```python
from build123d import *

# Parameters (mm, degrees)
F0_W     = 6.5
F0_H     = 9.5
F0_W_2   = 2
F0_H_2   = 13.4
F0_W_3   = 15.45
F0_H_3   = 16.4
F0_W_4   = 18.45
F0_H_4   = 0.8
F1_DEPTH = 1
F2_DEPTH = 3.5
F3_START = 3.5
F0_H_5   = 0.225
F3_DEPTH = 4.2
F4_DEPTH = 2.5


with BuildPart() as f1:
    # F0 (on Top) → F1 (new body)
    with BuildSketch(Plane.XY):
        with Locations((3.25, -9)):
            Rectangle(F0_W, F0_H)
        with Locations((43.5, -7.5)):
            Rectangle(F0_W_2, F0_H_2)
        Polygon((45, 0), (42.5, 0), (42.5, -0.8), (44.5, -0.8), (44.5, -14.2), (45, -14.2), align=None)
        with Locations((16.325, -9)):
            Rectangle(F0_W_3, F0_H_3)
        Polygon((42.5, -0.8), (24.05, -0.8), (24.05, -17.2), (42.5, -17.2), (42.5, -14.2), align=None)
        with Locations((33.275, -0.4)):
            Rectangle(F0_W_4, F0_H_4)
        Polygon((24.05, 0), (0, 0), (0, -4.25), (6.5, -4.25), (6.5, -13.75), (0, -13.75), (0, -18), (24.05, -18), (24.05, -17.2), (8.6, -17.2), (8.6, -0.8), (24.05, -0.8), align=None)
        with Locations((33.275, -17.6)):
            Rectangle(F0_W_4, F0_H_4)
    extrude(amount=F1_DEPTH)

    # F0 (on Top) → F2 (join)
    with BuildSketch(Plane.XY):
        with Locations((16.325, -9)):
            Rectangle(F0_W_3, F0_H_3)
        Polygon((42.5, -0.8), (24.05, -0.8), (24.05, -17.2), (42.5, -17.2), (42.5, -14.2), align=None)
        with Locations((43.5, -7.5)):
            Rectangle(F0_W_2, F0_H_2)
    extrude(amount=F2_DEPTH)

    # F0 (on Top) → F3 (join)
    with BuildSketch(Plane.XY.offset(F3_START)):
        with Locations((33.275, -0.4)):
            Rectangle(F0_W_4, F0_H_4)
        with Locations((33.275, 0.1125)):
            Rectangle(F0_W_4, F0_H_5)
        Polygon((42.5, -0.8), (24.05, -0.8), (24.05, -17.2), (42.5, -17.2), (42.5, -14.2), align=None)
        with Locations((33.275, -17.6)):
            Rectangle(F0_W_4, F0_H_4)
        with Locations((33.275, -18.1125)):
            Rectangle(F0_W_4, F0_H_5)
    extrude(amount=F3_DEPTH)

    # F0 (on Top) → F4 (join)
    with BuildSketch(Plane.XY):
        with Locations((3.25, -9)):
            Rectangle(F0_W, F0_H)
    extrude(amount=F4_DEPTH)


solid = f1.part
```
Geometry: final body of the model. Coordinates: model frame, mm. A direction names the side the tool comes from. Coordinates: 2 decimals unless noted, no trailing zeros. Order: outer loops, then holes, each group sorted by start corner. A loop starts at its lowest first (then second) coordinate and runs counter-clockwise, first axis right, second up. Notation, with made-up numbers: (51.5, 19) - (78.5, 19) arc R9 ccw to (78.5, 31) - close; hole circle Ø10 at (-2.5, -31). An arc over 180 degrees is marked (long way). Return JSON: item names as keys, results as strings. Group by question number.
1. Set-up query: faces 4 (the face through (3, -9, 2.5)), 5 (the face through (25, -17.2, 2)), 6 (the face through (44.5, -8, 2)), 7 (the face through (6.5, -9, 2)). Return all of +Z, -Z, +X, -X, +Y, -Y with unobstructed straight access to the full face (end or side cutting, diameter ignored); none if empty.
2. Cut plane D-D (z = 6). Output: boundary loops of the cut face in (x, y) (3 decimals), plus the area to 3 significant figures.
3. Material intervals for line 1 along X through (y, z) = (-8.75, 2.25); line 2 along Y through (x, z) = (13.5, 1.25); line 3 along X through (y, z) = (-16.5, 3.25), sorted ascending. Write a range as [from, to].
4. Pull-direction query (Z, two-part tool) for faces 1 (the face through (22, -9, 0)), 2 (the face through (7, -9, 1)), 3 (the face through (8.6, -9, 2)); classes: pulls with the +Z half, pulls with the -Z half, needs draft (parallel to the pull), parting line crosses it, or undercut.
5. Cut plane C-C (y = -13.25). Output: boundary loops of the cut face in (x, z), plus the area to 3 significant figures.
6. Pin query (flat end, axial travel): pin 1 (1.5 mm diameter, centred on y = -7, z = 6.5, fed in from -X); pin 2 (1 mm diameter, centred on x = 33, z = 2.5, fed in from +Y); pin 3 (5 mm diameter, centred on x = 2, y = -11, fed in from +Z). Return the tip coordinate at first contact, or that it passes through.
7. Cut plane B-B (x = 9). Output: boundary loops of the cut face in (y, z).
8. Cut plane A-A (z = 2). Output: boundary loops of the cut face in (x, y), plus the area to 3 significant figures.
Resolved:
{
 "1": {"face 4": "+Z, -X, +Y, -Y", "face 5": "+X, -X, -Y", "face 6": "+Z, +X, +Y, -Y", "face 7": "+Z, +Y, -Y"},
 "2": {"outline": "(24.05, -18.225) - (42.5, -18.225) - (42.5, 0.225) - (24.05, 0.225) - close", "area": "340 mm²"},
 "3": {"line 1": "x = [0, 6.5], [8.6, 44.5]", "line 2": "y = [-17.2, -0.8]", "line 3": "x = [8.6, 42.5]"},
 "4": {"face 1": "pulls with the -Z half", "face 2": "undercut", "face 3": "needs draft"},
 "5": {"outline": "(0, 0) - (45, 0) - (45, 1) - (44.5, 1) - (44.5, 3.5) - (42.5, 3.5) - (42.5, 7.7) - (24.05, 7.7) - (24.05, 3.5) - (8.6, 3.5) - (8.6, 1) - (6.5, 1) - (6.5, 2.5) - (0, 2.5) - close", "area": "222 mm²"},
 "6": {"pin 1": "stops at x = 24.05", "pin 2": "stops at y = -0.8", "pin 3": "stops at z = 2.5"},
 "7": {"outline": "(-18, 0) - (0, 0) - (0, 1) - (-0.8, 1) - (-0.8, 3.5) - (-17.2, 3.5) - (-17.2, 1) - (-18, 1) - close"},
 "8": {"outline": "(0, -13.75) - (6.5, -13.75) - (6.5, -4.25) - (0, -4.25) - close; (8.6, -17.2) - (42.5, -17.2) - (42.5, -14.2) - (44.5, -14.2) - (44.5, -0.8) - (8.6, -0.8) - close", "area": "645 mm²"}
}
